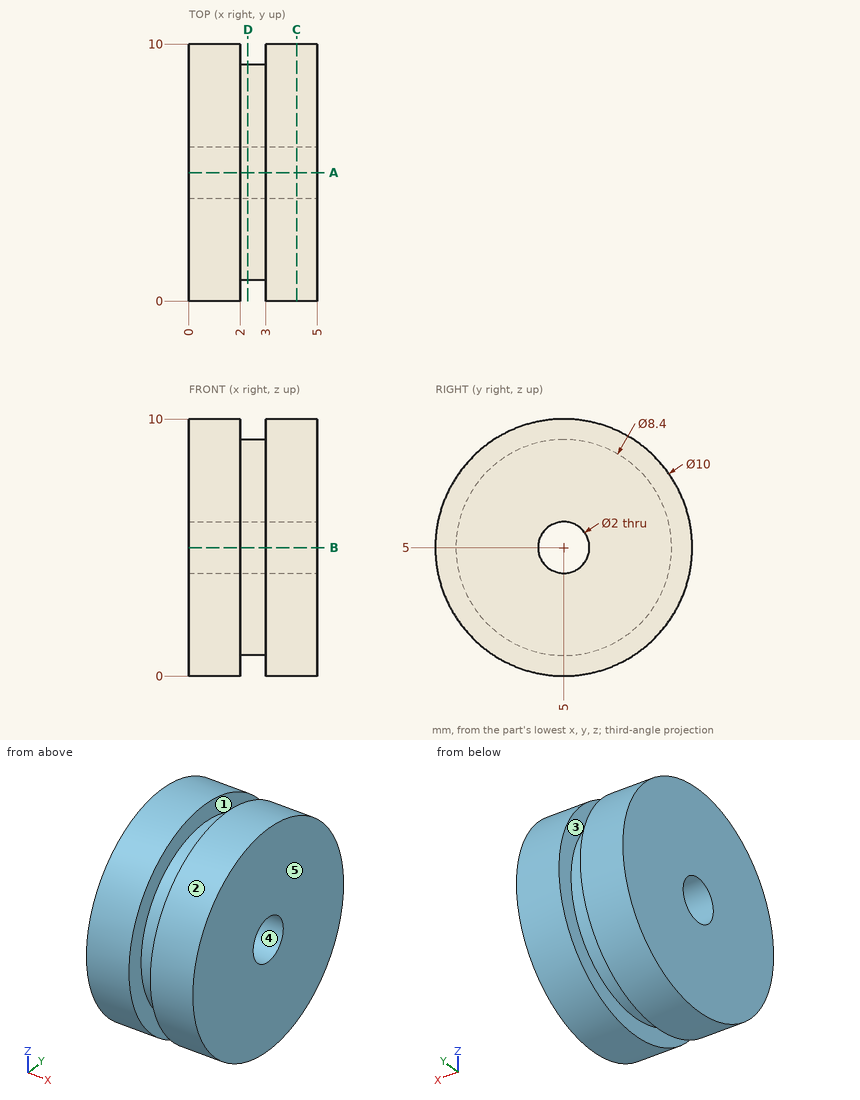
The figure shows three views and two pictorial views of one solid part (mm, origin at its lowest corner). Answer the questions. A direction names the side the tool comes from. Give positions to 0.01 mm unless a question says otherwise; leave off trailing zeros. Write each loop counter-clockwise with the first axis right and the second up, starting at its lowest first coordinate (ties: lowest second). Pieces come first, ordered by that corner, then holes.
Q1. The part is cut by section D-D on x = 2.3. Give the vertices of the cut face in (y, z), and give its area (3 significant figures).
Answer:
outline: circle Ø8.4 at (5, 5); hole circle Ø2 at (5, 5)
area: 52.3 mm2
Q2. Given pin 1 (1.5 mm diameter, centred on x = 1, y = 4, fed in from -Z); pin 2 (3 mm diameter, centred on x = 1, y = 8, fed in from -Z), each flat-ended and moving along its own axis, determine where each tip first touches the part or whether it passes through.
Answer:
pin 1: stops at z = 0.01
pin 2: stops at z = 0.23
Q3. For a pull along X with two mould halves and no side action, classify the marked faces 3, 4 and 5 as released by +X, released by -X, zero draft, split by the parting line, or undercut.
Answer:
face 3: undercut
face 4: zero draft
face 5: released by +X
Q4. A tool of negligible diameter and unlimited length cuts with its end or side. For the marked faces 1 and 2, from which of +Z, -Z, +X, -X, +Y, -Y can it reach the whole face along a straight path? Write none if from no direction.
Answer:
face 1: none
face 2: +X, -X
Q5. Straight lines are drawn through the part: L1, parallel to Z at x = 2.45, y = 5; L2, parallel to Z at x = 3.15, y = 5; L3, parallel to Z at x = 0.9, y = 9. For each, find the intervals that lie inside material, in ascending order.
Answer:
L1: z = 0.8 to 4, 6 to 9.2
L2: z = 0 to 4, 6 to 10
L3: z = 2 to 8
Q6. The part is cut by section C-C on x = 4.2. Give the vertices of the cut face in (y, z).
Answer:
outline: circle Ø10 at (5, 5); hole circle Ø2 at (5, 5)
Q7. The part is cut by section A-A on y = 5. Give the vertices of the cut face in (x, z), and give its area (3 significant figures).
Answer:
outline: (0, 0) - (2, 0) - (2, 0.8) - (3, 0.8) - (3, 0) - (5, 0) - (5, 4) - (0, 4) - close; (0, 6) - (5, 6) - (5, 10) - (3, 10) - (3, 9.2) - (2, 9.2) - (2, 10) - (0, 10) - close
area: 38.4 mm2
